Design review of the part built by this model. Coordinates are the model's own, in mm. A direction names the side the tool comes from. Round coordinates to 2 decimals unless told otherwise and drop trailing zeros. Order: outer loops, then holes, each group sorted by start corner. A loop starts at its lowest first (then second) coordinate and runs counter-clockwise, first axis right, second up. Notation, with made-up numbers: (-23, 79.5) - (19, 79.5) arc R16 ccw to (19, 85.5) - close; hole circle Ø6 at (44.5, 60). An arc over 180 degrees is marked (long way). Use CSV: the item, a comma, the result in double quotes. Start each with the question number.
from build123d import *

# Parameters (mm, degrees)
F0_W      = 67.2008618712
F0_H      = 151.4808684587
F0_R      = 10.082645717
F0_R_2    = 11.3219801377
F1_DEPTH  = 27.178
F2_W      = 43.0387500674
F2_H      = 97.4754467607
F3_DEPTH  = 68.326
F4_W      = 48.377899453
F4_H      = 38.2418624678
F5_DEPTH  = 120.904
F7_DEPTH  = 22.352
F8_DEPTH  = 1.016
F10_DEPTH = 25.908
F11_R     = 10.7410584699
F12_DEPTH = 138.938


with BuildPart() as f1:
    # F0 (on Top) → F1 (new body)
    with BuildSketch(Plane.XY):
        with Locations((0.662881881, 0.175178051)):
            Rectangle(F0_W, F0_H)
        with BuildLine():
            ThreePointArc((34.2633128166, 75.9156122804), (0.662881881, 109.516043216), (-32.9375490546, 75.9156122804))
            Line((-32.9375490546, 75.9156122804), (34.2633128166, 75.9156122804))
        make_face()
        with Locations((0, 92.8106307983)):
            Circle(F0_R, mode=Mode.SUBTRACT)
        with BuildLine():
            Line((34.2633128166, -75.5652561784), (-32.9375490546, -75.5652561784))
            ThreePointArc((-32.9375490546, -75.5652561784), (0.662881881, -109.165687114), (34.2633128166, -75.5652561784))
        make_face()
        with Locations((0, -91.1173969507)):
            Circle(F0_R_2, mode=Mode.SUBTRACT)
    extrude(amount=F1_DEPTH)

    # F2 (on face) → F3 (join)
    with BuildSketch(Plane.XY.offset(27.178)):
        with Locations((-0.206517987, 4.2744092643)):
            Rectangle(F2_W, F2_H)
    extrude(amount=F3_DEPTH)

    # F4 (on face) → F5 (cut)
    with BuildSketch(Plane.YZ.offset(21.3128570467)):
        with Locations((5.5104782805, 76.3830687661)):
            Rectangle(F4_W, F4_H)
        with BuildLine():
            Line((29.699428007, 57.2621375322), (-18.678471446, 57.2621375322))
            ThreePointArc((-18.678471446, 57.2621375322), (5.5104782805, 33.0731878057), (29.699428007, 57.2621375322))
        make_face()
    extrude(amount=-F5_DEPTH, mode=Mode.SUBTRACT)

    # F6 (on face) → F7 (join)
    with BuildSketch(Plane(origin=(0, 53.0121326447, 0), x_dir=(-1, 0, 0), z_dir=(0, 1, 0))):
        with BuildLine():
            Line((-21.3128570467, 95.504), (21.7258930206, 95.504))
            ThreePointArc((21.7258930206, 95.504), (0.206517987, 117.0233750337), (-21.3128570467, 95.504))
        make_face()
    extrude(amount=-F7_DEPTH)

    # F8 (add): a face of the model
    f8_faces = [f1.faces().sort_by_distance(p)[0] for p in [
        (-0.206517987, 30.6601326447, 104.6371064236),
    ]]
    extrude(f8_faces, amount=F8_DEPTH)

    # F9 (on face) → F10 (join)
    with BuildSketch(Plane.XZ.offset(44.463314116)):
        with BuildLine():
            Line((-21.7258930206, 95.504), (21.3128570467, 95.504))
            ThreePointArc((21.3128570467, 95.504), (-0.206517987, 117.0233750337), (-21.7258930206, 95.504))
        make_face()
    extrude(amount=-F10_DEPTH)

    # F11 (on face) → F12 (cut)
    with BuildSketch(Plane.XZ.offset(44.463314116)):
        with Locations((-0.206517987, 95.504)):
            Circle(F11_R)
    extrude(amount=-F12_DEPTH, mode=Mode.SUBTRACT)


solid = f1.part
Q1. The part is to be moulded in two halves that separate along Z. For faces 3 (the cylindrical face through (-1.605, -31.691, 106.154)), 4 (the flat face through (-22, 2, 27.178)), 5 (the flat face through (-1, -44.463, 63)), say which applies: +Z half, -Z half, draft (parallel to the pull), parting line (faces both ways), or undercut.
Q2. Clearance check with flat-ended pins moving along their axes: pin 1 (3 mm diameter, centred on x = -13, z = 23, fed in from -Y); pin 2 (5 mm diameter, centred on x = -21.5, z = 24, fed in from -Y); pin 3 (20 mm diameter, centred on x = 14.5, y = -47, fed in from +Z). State where each tip first meets the part, or that it passes through.
Q3. Take a section at D-D (y = -64.5). State the section outline as (x, z) points, plus the area to 3 significant figures.
Q4. For L1, parallel to Y at x = 0, z = 17; L2, parallel to Y at x = 21, z = 66; L3, parallel to Z at x = -28, y = 90, list the stretches that pass through material, from the lowest coordinate up. Write a range as [from, to].
Q5. Take a section at C-C (z = 103.5). State the section outline as (x, y) points.
Q6. Take a section at B-B (x = 0). State the section outline as (y, z) points.
Q7. Take a section at A-A (z = 69). State the section outline as (x, y) points, plus the area to 3 significant figures.
Q8. Tool access review of faces 1 (the flat face through (0, 53.012, 63)), 2 (the flat face through (-32.938, -1, 13)): name each direction out of +Z, -Z, +X, -X, +Y, -Y from which nothing blocks a thin tool from reaching the whole face with its end or side.
Findings below:
1,face 3,"undercut"
1,face 4,"+Z half"
1,face 5,"draft"
2,pin 1,"stops at y = -106.89"
2,pin 2,"stops at y = -102.81"
2,pin 3,"stops at z = 116.43"
3,outline,"(-32.94, 0) - (34.26, 0) - (34.26, 27.18) - (-32.94, 27.18) - close"
3,area,"1,830 mm^2"
4,L1,"y = [-109.16, -102.44], [-79.8, 82.73], [102.89, 109.51]"
4,L2,"y = [-44.46, -18.68], [29.7, 53.01]"
4,L3,"z = [0, 27.18]"
5,outline,"(-20.19, -44.46) - (-7.38, -44.46) - (-7.38, -18.56) - (-20.19, -18.56) - close; (-20.19, 29.64) - (-7.38, 29.64) - (-7.38, 53.01) - (-20.19, 53.01) - close; (6.97, -44.46) - (19.77, -44.46) - (19.77, -18.56) - (6.97, -18.56) - close; (6.97, 29.64) - (19.77, 29.64) - (19.77, 53.01) - (6.97, 53.01) - close"
6,outline,"(-109.16, 0) - (-102.44, 0) - (-102.44, 27.18) - (-109.16, 27.18) - close; (-79.8, 0) - (82.73, 0) - (82.73, 27.18) - (53.01, 27.18) - (53.01, 84.76) - (29.7, 84.76) - (29.7, 57.26) arc R24.19 cw to (-18.68, 57.26) - (-18.68, 84.76) - (-44.46, 84.76) - (-44.46, 27.18) - (-79.8, 27.18) - close; (-44.46, 106.24) - (-18.56, 106.24) - (-18.56, 117.02) - (-44.46, 117.02) - close; (29.64, 106.24) - (53.01, 106.24) - (53.01, 117.02) - (29.64, 117.02) - close; (102.89, 0) - (109.51, 0) - (109.51, 27.18) - (102.89, 27.18) - close"
7,outline,"(-21.73, -44.46) - (21.31, -44.46) - (21.31, -18.68) - (-21.73, -18.68) - close; (-21.73, 29.7) - (21.31, 29.7) - (21.31, 53.01) - (-21.73, 53.01) - close"
7,area,"2,110 mm^2"
8,face 1,"+Z, +X, -X, +Y"
8,face 2,"+Z, -Z, -X, +Y, -Y"
